Geometry check sheet. Reference: the model listing, model coordinates, mm. Coordinates: 2 decimals unless noted, no trailing zeros. Write each loop counter-clockwise with the first axis right and the second up, starting at its lowest first coordinate (ties: lowest second). Pieces come first, ordered by that corner, then holes. Notation, with made-up numbers: M 10.25,44 L 61.25,44 A16 cw 61.25,71 Z; hole C 79.5,74.25 d8. An arc over 180 degrees is marked long. Write each question's results on one line, items separated by ' | '.
```python
from build123d import *

# Parameters (mm, degrees)
SKETCH2_W           = 241.3
SKETCH2_H           = 133.35
BOSS_EXTRUDE1_DEPTH = 6.35
SKETCH3_W           = 6.35
SKETCH3_H           = 12.7
CUT_EXTRUDE1_DEPTH  = 7.35
LPATTERN1_COUNT     = 6
LPATTERN1_PITCH     = 25.4
SKETCH4_W           = 12.7
SKETCH4_H           = 6.35
CUT_EXTRUDE2_DEPTH  = 7.35
LPATTERN2_COUNT     = 10
LPATTERN2_PITCH     = 25.4
SKETCH5_W           = 12.7
SKETCH5_H           = 6.35
CUT_EXTRUDE3_DEPTH  = 7.35
LPATTERN3_COUNT     = 10
LPATTERN3_PITCH     = 25.4
SKETCH6_W           = 203.2
SKETCH6_H           = 95.25
CUT_EXTRUDE4_DEPTH  = 7.35
FILLET1_R           = 25.4


with BuildPart() as part:
    # Sketch2 → Boss-Extrude1 (new body)
    with BuildSketch(Plane(origin=(0, 0, 0), x_dir=(1, 0, 0), z_dir=(0, 1, 0))):
        with Locations((120.65, 66.675)):
            Rectangle(SKETCH2_W, SKETCH2_H)
    extrude(amount=BOSS_EXTRUDE1_DEPTH)

    # Sketch3 → Cut-Extrude1 (cut, through all)
    with BuildSketch(Plane(origin=(0, 6.35, 0), x_dir=(1, 0, 0), z_dir=(0, 1, 0))):
        with Locations((3.175, 6.35)):
            Rectangle(SKETCH3_W, SKETCH3_H)
        with Locations((238.125, 6.35)):
            Rectangle(SKETCH3_W, SKETCH3_H)
    cut_extrude1 = extrude(amount=-CUT_EXTRUDE1_DEPTH, mode=Mode.SUBTRACT)

    # LPattern1: Cut-Extrude1 ×6
    with Locations(*[(0, 0, -i * LPATTERN1_PITCH) for i in range(1, LPATTERN1_COUNT)]):
        add(cut_extrude1, mode=Mode.SUBTRACT)

    # Sketch4 → Cut-Extrude2 (cut, through all)
    with BuildSketch(Plane(origin=(0, 6.35, 0), x_dir=(1, 0, 0), z_dir=(0, 1, 0))):
        with Locations((222.25, 3.175)):
            Rectangle(SKETCH4_W, SKETCH4_H)
    cut_extrude2 = extrude(amount=-CUT_EXTRUDE2_DEPTH, mode=Mode.SUBTRACT)

    # LPattern2: Cut-Extrude2 ×10
    with Locations(*[(-i * LPATTERN2_PITCH, 0, 0) for i in range(1, LPATTERN2_COUNT)]):
        add(cut_extrude2, mode=Mode.SUBTRACT)

    # Sketch5 → Cut-Extrude3 (cut, through all)
    with BuildSketch(Plane(origin=(0, 6.35, 0), x_dir=(1, 0, 0), z_dir=(0, 1, 0))):
        with Locations((6.35, 130.175)):
            Rectangle(SKETCH5_W, SKETCH5_H)
    cut_extrude3 = extrude(amount=-CUT_EXTRUDE3_DEPTH, mode=Mode.SUBTRACT)

    # LPattern3: Cut-Extrude3 ×10
    with Locations(*[(i * LPATTERN3_PITCH, 0, 0) for i in range(1, LPATTERN3_COUNT)]):
        add(cut_extrude3, mode=Mode.SUBTRACT)

    # Sketch6 → Cut-Extrude4 (cut, through all)
    with BuildSketch(Plane(origin=(0, 6.35, 0), x_dir=(1, 0, 0), z_dir=(0, 1, 0))):
        with Locations((120.65, 66.675)):
            Rectangle(SKETCH6_W, SKETCH6_H)
    extrude(amount=-CUT_EXTRUDE4_DEPTH, mode=Mode.SUBTRACT)

    # Fillet1
    fillet1_edges = [part.edges().sort_by_distance(p)[0] for p in [
        (19.05, 3.175, -19.05),
        (19.05, 3.175, -114.3),
        (222.25, 3.175, -114.3),
        (222.25, 3.175, -19.05),
    ]]
    fillet(fillet1_edges, radius=FILLET1_R)


solid = part.part
```
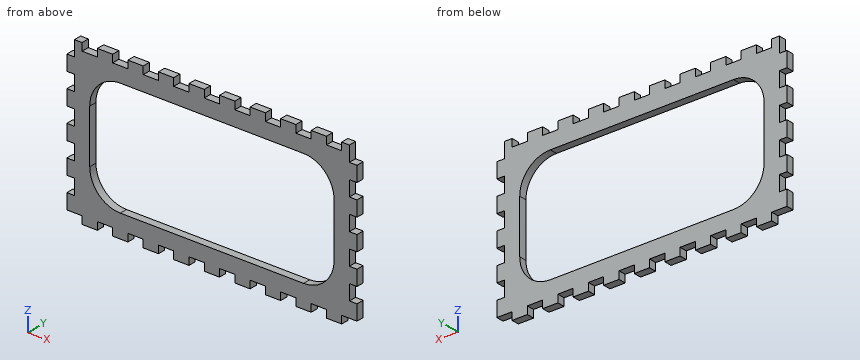
Q1. Sectioned sample at B-B on x = 148. Record the cut outline in (y, z), and give its area (3 significant figures).
Geometry check:
outline: M 0,-133.35 L 6.35,-133.35 L 6.35,-114.3 L 0,-114.3 Z; M 0,-19.05 L 6.35,-19.05 L 6.35,-6.35 L 0,-6.35 Z | area: 202 mm2
Q2. Depth check by flat-ended pin: P1, Ø1.9, axis at y = 2.5, z = -130, coming from the +X side; P2, Ø3, axis at y = 2, z = -4, coming from the +X side; P3, Ø3, axis at x = 173.5, y = 3.5, coming from the +Z side. Enter the tip coordinate at first touch or a pass-through.
Geometry check:
P1: stops at x = 228.6 | P2: stops at x = 234.95 | P3: stops at z = -6.35
Q3. Scan lines: probe 1 along X at (y, z) = (4.5, -75); probe 2 along Z at (x, y) = (186.5, 5.5); probe 3 along Z at (x, y) = (99.5, 6). Record each from-to range of solid material in increasing order.
Geometry check:
probe 1: x = 0 to 19.05, 222.25 to 241.3 | probe 2: z = -127 to -114.3, -19.05 to 0 | probe 3: z = -133.35 to -114.3, -19.05 to -6.35
Q4. Sectioned sample at A-A on z = -47. Record the cut outline in (x, y), and give its area (3 significant figures).
Geometry check:
outline: M 0,0 L 19.05,0 L 19.05,6.35 L 0,6.35 Z; M 222.25,0 L 241.3,0 L 241.3,6.35 L 222.25,6.35 Z | area: 242 mm2
